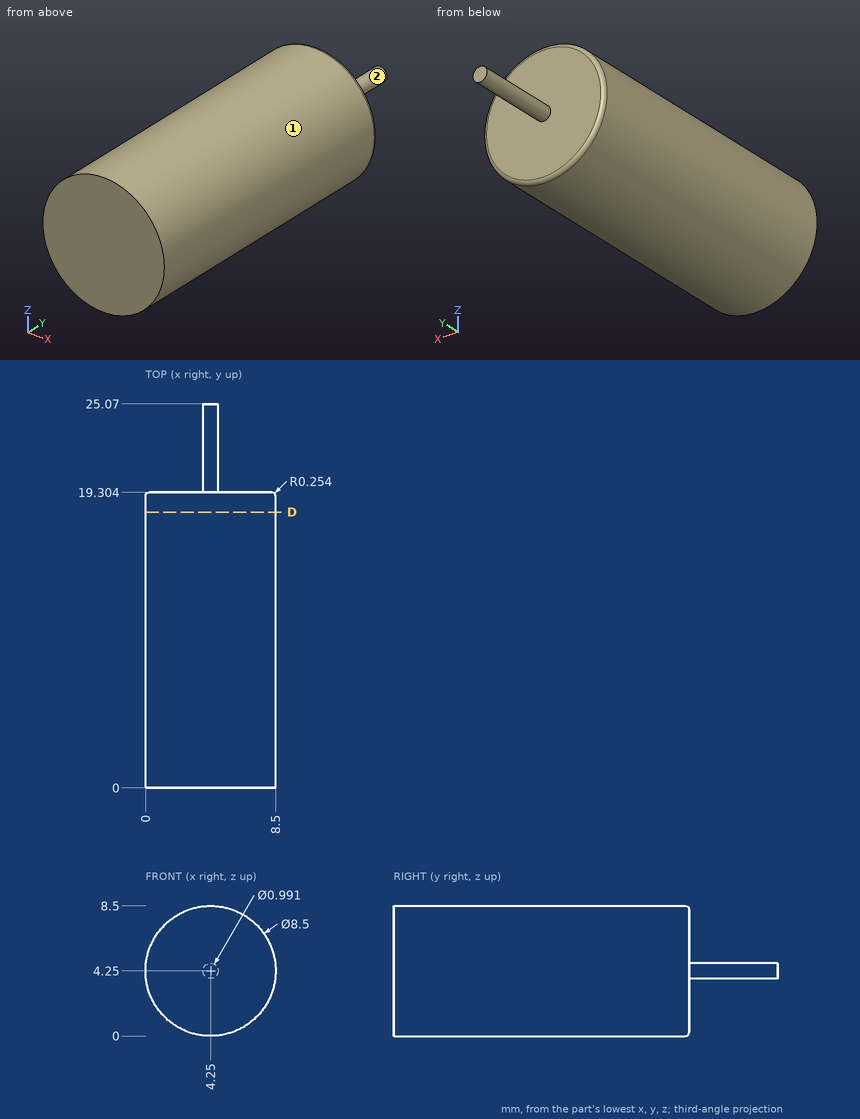
Print and shaded views of the part. All mm, measured from the part's lowest x, y and z. A direction names the side the tool comes from. Round coordinates to 2 decimals unless told otherwise and drop trailing zeros. Write each loop counter-clockwise with the first axis right and the second up, starting at its lowest first coordinate (ties: lowest second). Pieces come first, ordered by that corner, then holes. Notation, with made-up numbers: M 71.25,-31.75 L 84.25,-31.75 A24 cw 84.25,-15.75 Z; hole C 74,11 d6. An arc over 180 degrees is marked long. Use a Markdown table: item, result. Add a question column.
1. 3-axis set-ups, long thin cutter, end or side, ignore diameter. For the marked faces 1 and 2: which of +Z, -Z, +X, -X, +Y, -Y reach the whole face in a straight line?
2. Drill centre lines: probe 1 along Y at (x, z) = (3.5, 7.5); probe 2 along X at (y, z) = (16.75, 8); probe 3 along Z at (x, y) = (7.5, 6.25). Where is each one in solid material? Low to high.
3. Slice it at D-D on y = 18. Give the cut face in (x, z).
4. Flat gauge pins, fed straight in: P1, Ø2, axis at y = 18.5, z = 5.5, coming from the -X side; P2, Ø3, axis at y = 21.5, z = 3.5, coming from the +X side (1 decimal). Where does each tip first touch, or does it go through?
Reply:
| question | item | result |
|---|---|---|
| 1 | face 1 | +Y, -Y |
| 1 | face 2 | +Y |
| 2 | probe 1 | y = 0 to 19.3 |
| 2 | probe 2 | x = 2.25 to 6.25 |
| 2 | probe 3 | z = 1.51 to 6.99 |
| 3 | outline | C 4.25,4.25 d8.5 |
| 4 | P1 | stops at x = 0.01 |
| 4 | P2 | stops at x = 4.7 |
